Source: CAD feature listing. Evaluate the final solid. Frame: model axes, mm. Coordinates: 2 decimals unless noted, no trailing zeros. Loops run counter-clockwise (first coordinate to the right, second up) from the corner with the lowest first, then second, coordinate; pieces in that order, holes last. Notation, with made-up numbers: (79.5, -1) - (133.5, -1) arc R33 cw to (133.5, 35) - close; hole circle Ø8 at (71.25, -10.5). An arc over 180 degrees is marked (long way). Write item = value, one per line. Start each with the question number.
Autodesk Inventor part; units mm, degrees
ref_plane "YZ Plane" through (0, 0, 0) normal (1, 0, 0) x (0, 1, 0)
ref_plane "XZ Plane" through (0, 0, 0) normal (0, 1, 0) x (-1, 0, 0)
ref_plane "XY Plane" through (0, 0, 0) normal (0, 0, 1) x (1, 0, 0)
sketch "Sketch9" plane through (0, 0, 0) normal (0, 1, 0) x (-1, 0, 0)
  line L0 (20, 10) -> (-20, 10)
  line L1 (-20, 10) -> (-20, -10)
  line L2 (-20, -10) -> (20, -10)
  line L3 (20, -10) -> (20, 10)
  line L4 (20, 10) -> (-20, -10) construction
  line L5 (-20, 10) -> (20, -10) construction
  line L6 (-18, 8) -> (18, 8)
  line L7 (18, 8) -> (18, -8)
  line L8 (18, -8) -> (-18, -8)
  line L9 (-18, -8) -> (-18, 8)
  point P0 (0, 0)
  dimension "d172" = 40
  dimension "d173" = 20
  dimension "d174" = 2
extrude "Extrusion3" add sketch "Sketch9" against normal blind 1200
sketch "Sketch10" plane through (0, 0, 0) normal (1, 0, 0) x (0, 1, 0)
  line L0 (0, 10) -> (0, -10) construction
  line L1 (0, 10) -> (-1200, 10) construction
  line L2 (-1200, -10) -> (-1200, 10) construction
  line L3 (0, -10) -> (-1200, -10) construction
  line L4 (-148.5, 8.5) -> (-131.5, 8.5)
  line L5 (-131.5, 8.5) -> (-131.5, -8.5)
  line L6 (-131.5, -8.5) -> (-148.5, -8.5)
  line L7 (-148.5, -8.5) -> (-148.5, 8.5)
  line L8 (-148.5, 8.5) -> (-131.5, -8.5) construction
  line L9 (-131.5, 8.5) -> (-148.5, -8.5) construction
  line L10 (-308.5, 8.5) -> (-291.5, 8.5)
  line L11 (-291.5, 8.5) -> (-291.5, -8.5)
  line L12 (-291.5, -8.5) -> (-308.5, -8.5)
  line L13 (-308.5, -8.5) -> (-308.5, 8.5)
  line L14 (-308.5, 8.5) -> (-291.5, -8.5) construction
  line L15 (-291.5, 8.5) -> (-308.5, -8.5) construction
  line L16 (-428.5, 8.5) -> (-411.5, 8.5)
  line L17 (-411.5, 8.5) -> (-411.5, -8.5)
  line L18 (-411.5, -8.5) -> (-428.5, -8.5)
  line L19 (-428.5, -8.5) -> (-428.5, 8.5)
  line L20 (-428.5, 8.5) -> (-411.5, -8.5) construction
  line L21 (-411.5, 8.5) -> (-428.5, -8.5) construction
  circle A0 centre (-470, 0) radius 8.5
  line L22 (0, 0) -> (30, 0)
  circle A1 centre (-140, 0) radius 8.5
  circle A2 centre (-300, 0) radius 8.5
  circle A3 centre (-420, 0) radius 8.5
  dimension "d177" = 17
  dimension "d178" = 17
  dimension "d181" = 30
  dimension "d182" = 170
  dimension "d183" = 330
  dimension "d184" = 450
  dimension "d185" = 500
  dimension "d186" = 17
extrude "Extrusion4" [suppressed]
properties part number "TKS 3562 FDS support tube" material "Stainless Steel"
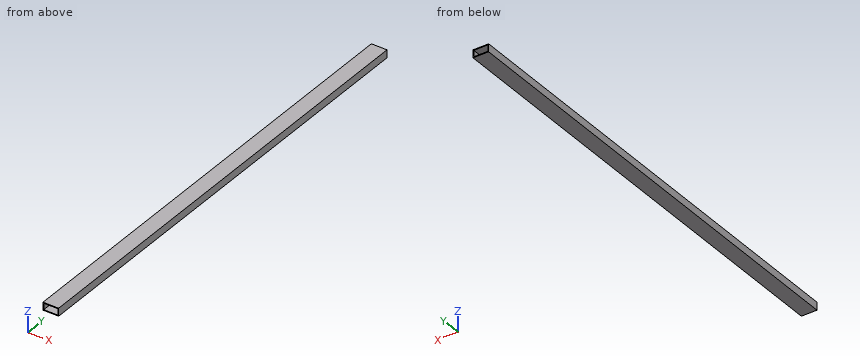
Item 1: Cut plane A-A (z = -0.5). Return the cut outline in (x, y).
Item 2: Cut plane B-B (y = -909). Return the cut outline in (x, z), then the cut area to 3 significant figures.
Item 3: Cut plane C-C (x = -8). Return the cut outline in (y, z), then the cut area to 3 significant figures.
Item 4: Material intervals for L1, parallel to Z at x = 16, y = -563.5; L2, parallel to X at y = -806, z = -1.5, sorted ascending. Write a range as [from, to].
Responses:
q1.outline = (-20, -1200) - (-18, -1200) - (-18, 0) - (-20, 0) - close; (18, -1200) - (20, -1200) - (20, 0) - (18, 0) - close
q2.outline = (-20, -10) - (20, -10) - (20, 10) - (-20, 10) - close; hole (-18, -8) - (18, -8) - (18, 8) - (-18, 8) - close
q2.area = 224 mm2
q3.outline = (-1200, -10) - (0, -10) - (0, -8) - (-1200, -8) - close; (-1200, 8) - (0, 8) - (0, 10) - (-1200, 10) - close
q3.area = 4,800 mm2
q4.L1 = [-10, -8], [8, 10]
q4.L2 = [-20, -18], [18, 20]
